Design review of the part built by this model. Coordinates are the model's own, in mm. A direction names the side the tool comes from. Coordinates: 2 decimals unless noted, no trailing zeros. Write each loop counter-clockwise with the first axis right and the second up, starting at its lowest first coordinate (ties: lowest second). Pieces come first, ordered by that corner, then holes. Notation, with made-up numbers: M -4,86 L 23,86 A20 ccw 23,99 Z; hole C 71,9.25 d5. An arc over 180 degrees is marked long. Return JSON: item names as keys, results as strings. Group by question number.
```python
from build123d import *

# Parameters (mm, degrees)
SKETCH_1_W          = 110
SKETCH_1_H          = 110
EXTRUDE_1_DEPTH     = 38
SKETCH_3_W          = 104
SKETCH_3_H          = 104
CUT_EXTRUDE_1_DEPTH = 32
FILLET_1_R          = 3
FILLET_2_R          = 3
CUT_EXTRUDE_2_DEPTH = 85.107074613
FILLET_3_R          = 3
CUT_EXTRUDE_4_DEPTH = 1
CUT_EXTRUDE_5_DEPTH = 3
SKETCH_13_W         = 104
SKETCH_13_H         = 104
CUT_EXTRUDE_6_DEPTH = 3


with BuildPart() as part:
    # 草图1 → 凸台-拉伸1 (new body)
    with BuildSketch(Plane.XY):
        Rectangle(SKETCH_1_W, SKETCH_1_H)
    extrude(amount=EXTRUDE_1_DEPTH)

    # 草图3 → 切除-拉伸1 (cut)
    with BuildSketch(Plane.XY.offset(38)):
        Rectangle(SKETCH_3_W, SKETCH_3_H)
    extrude(amount=-CUT_EXTRUDE_1_DEPTH, mode=Mode.SUBTRACT)

    # 圆角1
    fillet_1_edges = [part.edges().sort_by_distance(p)[0] for p in [
        (55, -55, 19),
        (55, 55, 19),
    ]]
    fillet(fillet_1_edges, radius=FILLET_1_R)

    # 圆角2
    fillet_2_edges = [part.edges().sort_by_distance(p)[0] for p in [
        (-55, 55, 19),
        (-55, -55, 19),
    ]]
    fillet(fillet_2_edges, radius=FILLET_2_R)

    # 草图4 → 切除-拉伸2 (cut, through all)
    with BuildSketch(Plane.XY.offset(6)):
        with BuildLine():
            Line((-3.909141934, -47.255379726), (3.909141934, -47.255379726))
            ThreePointArc((3.909141934, -47.255379726), (5.159141934, -48.505379726), (3.909141934, -49.755379726))
            Line((3.909141934, -49.755379726), (-3.909141934, -49.755379726))
            ThreePointArc((-3.909141934, -49.755379726), (-5.159141934, -48.505379726), (-3.909141934, -47.255379726))
        make_face()
    extrude(amount=-CUT_EXTRUDE_2_DEPTH, mode=Mode.SUBTRACT)

    # 圆角3
    fillet_3_edges = [part.edges().sort_by_distance(p)[0] for p in [
        (55, 0, 0),
        (54.121320344, 54.121320344, 0),
        (54.121320344, -54.121320344, 0),
        (0, -55, 0),
        (-55, 0, 0),
        (0, 55, 0),
        (-54.121320344, 54.121320344, 0),
        (-54.121320344, -54.121320344, 0),
    ]]
    fillet(fillet_3_edges, radius=FILLET_3_R)

    # 草图7 → 切除-拉伸4 (cut)
    with BuildSketch(Plane(origin=(0, 0, 0), x_dir=(-1, 0, 0), z_dir=(0, 0, -1))):
        with BuildLine():
            Line((27.351581896, -16.692025534), (72.045241502, -16.692025534))
            ThreePointArc((72.045241502, -16.692025534), (78.315018535, -22.961802567), (72.045241502, -29.231579599))
            Line((72.045241502, -29.231579599), (27.351581896, -29.231579599))
            ThreePointArc((27.351581896, -29.231579599), (21.081804864, -22.961802567), (27.351581896, -16.692025534))
        make_face()
        with BuildLine():
            Line((27.389277991, -35.286565578), (72.382937597, -35.286565578))
            ThreePointArc((72.382937597, -35.286565578), (78.652714629, -41.556342611), (72.382937597, -47.826119643))
            Line((72.382937597, -47.826119643), (27.389277991, -47.826119643))
            ThreePointArc((27.389277991, -47.826119643), (21.119500958, -41.556342611), (27.389277991, -35.286565578))
        make_face()
        with BuildLine():
            Line((26.949815907, -0.968873845), (71.943475513, -0.968873845))
            ThreePointArc((71.943475513, -0.968873845), (78.213252546, -7.238650877), (71.943475513, -13.50842791))
            Line((71.943475513, -13.50842791), (26.949815907, -13.50842791))
            ThreePointArc((26.949815907, -13.50842791), (20.680038875, -7.238650877), (26.949815907, -0.968873845))
        make_face()
        with BuildLine():
            Line((-74.834862022, -16.710464099), (-29.841202416, -16.710464099))
            ThreePointArc((-29.841202416, -16.710464099), (-23.571425383, -22.980241131), (-29.841202416, -29.250018164))
            Line((-29.841202416, -29.250018164), (-74.834862022, -29.250018164))
            ThreePointArc((-74.834862022, -29.250018164), (-81.104639054, -22.980241131), (-74.834862022, -16.710464099))
        make_face()
        with BuildLine():
            Line((-74.497165928, -35.305004142), (-29.503506322, -35.305004142))
            ThreePointArc((-29.503506322, -35.305004142), (-23.233729289, -41.574781175), (-29.503506322, -47.844558208))
            Line((-29.503506322, -47.844558208), (-74.497165928, -47.844558208))
            ThreePointArc((-74.497165928, -47.844558208), (-80.76694296, -41.574781175), (-74.497165928, -35.305004142))
        make_face()
        with BuildLine():
            Line((-74.936628011, -0.987312409), (-29.942968405, -0.987312409))
            ThreePointArc((-29.942968405, -0.987312409), (-23.673191373, -7.257089442), (-29.942968405, -13.526866474))
            Line((-29.942968405, -13.526866474), (-74.936628011, -13.526866474))
            ThreePointArc((-74.936628011, -13.526866474), (-81.206405044, -7.257089442), (-74.936628011, -0.987312409))
        make_face()
    extrude(amount=-CUT_EXTRUDE_4_DEPTH, mode=Mode.SUBTRACT)

    # 草图10 → 切除-拉伸5 (cut)
    with BuildSketch(Plane(origin=(0, 0, 0), x_dir=(-1, 0, 0), z_dir=(0, 0, -1))):
        with BuildLine():
            Line((-3.558455997, -46.531518088), (4.441544003, -46.531518088))
            ThreePointArc((4.441544003, -46.531518088), (6.466487551, -48.556461636), (4.441544003, -50.581405184))
            Line((4.441544003, -50.581405184), (-3.558455997, -50.581405184))
            ThreePointArc((-3.558455997, -50.581405184), (-5.583399545, -48.556461636), (-3.558455997, -46.531518088))
        make_face()
    extrude(amount=-CUT_EXTRUDE_5_DEPTH, mode=Mode.SUBTRACT)

    # 草图13 → 切除-拉伸6 (cut)
    with BuildSketch(Plane.XY.offset(6)):
        Rectangle(SKETCH_13_W, SKETCH_13_H)
    extrude(amount=-CUT_EXTRUDE_6_DEPTH, mode=Mode.SUBTRACT)


solid = part.part
```
Item 1: Machinability: for faces 4 (the flat face through (-1, 1, 3)), 5 (the flat face through (0, -50.581, 1)), 6 (the flat face through (39, -23, 1)), 7 (the cylindrical face through (-21.12, -41.69, 0.49)), which of the approach directions +Z, -Z, +X, -X, +Y, -Y give a long, thin tool a straight path to every point of the face, cutting with its end or side? Answer none if there is none.
Item 2: Add section A-A (z = 4.5). Write out the cut boundary in (x, y).
Item 3: Add section C-C (x = -33.5). Write out the cut boundary in (y, z), plus the area to 3 significant figures.
Item 4: For line 1 (Y direction, x = -49.5, z = 32); line 2 (Z direction, x = 23, y = -5), list the stretches that pass through material, from the lowest coordinate up.
Item 5: The part is to be moulded in two halves that separate along Y. For faces 1 (the flat face through (-1, 12, 0)), 2 (the flat face through (-1, -55, 20)), 3 (the cylindrical face through (23.235, -41.437, 0.493)), say which applies: pulls with the +Y half, pulls with the -Y half, needs draft (parallel to the pull), parting line crosses it, or undercut.
Item 6: Add section B-B (y = 0.5). Write out the cut boundary in (x, z).
Item 7: For pin 1 (0.8 mm diameter, centred on x = -47, z = 0.5, fed in from +Y); pin 2 (1.5 mm diameter, centred on x = -0.5, z = 1, fed in from -Y); pin 3 (2.5 mm diameter, centred on x = -0.5, z = 1, fed in from +Y); pin 4 (14 mm diameter, centred on x = -30, y = -41, fed in from -Z), all flat-tipped, find the tip position at first contact; note any pin that passes through.
Geometry check:
{
 "1": {"face 4": "+Z", "face 5": "+Z, -Z", "face 6": "-Z, +X", "face 7": "-Z, -X"},
 "2": {"outline": "M -55,-52 A3 ccw -52,-55 L 52,-55 A3 ccw 55,-52 L 55,52 A3 ccw 52,55 L -52,55 A3 ccw -55,52 Z; hole M -52,-52 L 52,-52 L 52,52 L -52,52 Z"},
 "3": {"outline": "M -55,3 A3 ccw -52,0 L -47.83,0 L -47.83,1 L -35.29,1 L -35.29,0 L -29.23,0 L -29.23,1 L -16.69,1 L -16.69,0 L -13.51,0 L -13.51,1 L -0.97,1 L -0.97,0 L 52,0 A3 ccw 55,3 L 55,38 L 52,38 L 52,3 L -52,3 L -52,38 L -55,38 Z", "area": "499 mm^2"},
 "4": {"line 1": "-55 to -52, 52 to 55", "line 2": "0 to 3"},
 "5": {"face 1": "needs draft", "face 2": "pulls with the -Y half", "face 3": "undercut"},
 "6": {"outline": "M -55,3 A3 ccw -52,0 L 52,0 A3 ccw 55,3 L 55,38 L 52,38 L 52,3 L -52,3 L -52,38 L -55,38 Z"},
 "7": {"pin 1": "y = 54.14", "pin 2": "y = -54.73", "pin 3": "y = 54.9", "pin 4": "z = 0"}
}
